Study the drawing (mm; zero at the part's minimum x, y, z) and answer. A direction names the side the tool comes from. Coordinates: 2 decimals unless noted, no trailing zeros. Loops run counter-clockwise (first coordinate to the right, second up) from the corner with the lowest first, then second, coordinate; pieces in that order, holes last. Notation, with made-up numbers: (-26.75, -31) - (-0.75, -31) arc R18 ccw to (-0.75, -16) - close; hole circle Ø8 at (41.25, -28.5). An arc over 180 degrees is marked (long way). Use one line per item in the form item = value. Start each with the question number.
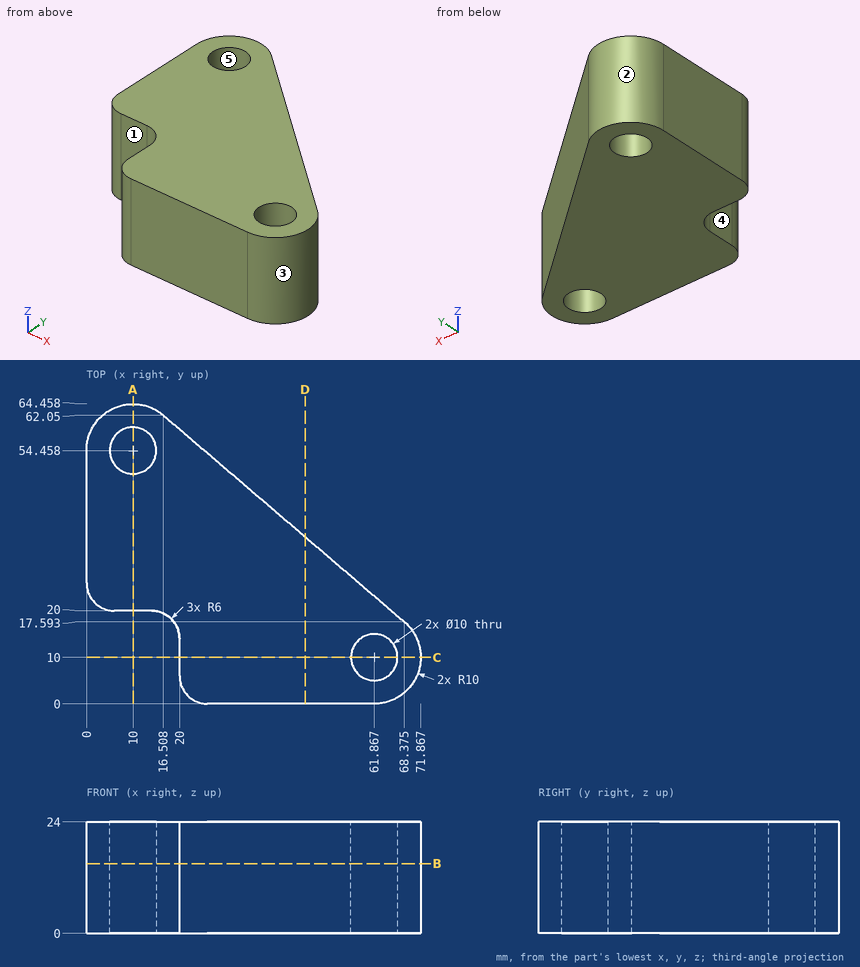
(1) For the marked faces 1 and 2, determine the directions among +Z, -Z, +X, -X, +Y, -Y from which every point of the face is accessible in a straight line to the end or side of a thin tool.
(2) Each of these flat-tipped pins is pushed along its axis until it touches: pin 1 Ø4 at (y, z) = (7, 3.5) entering from +X; pin 2 Ø16 at (x, y) = (61.87, 10) entering from -Z; pin 3 Ø9 at (x, z) = (11, 9) entering from -Y; pin 4 Ø6 at (x, y) = (10, 54.46) entering from +Z. Where does it stop, or does it pass through?
(3) A cutting plane is placed at A-A (x = 10). Determine the outline of the cut face in (y, z).
(4) Determine the mould class of the marked faces 3, 4 and 5 for opening direction Y: +Y half, -Y half, draft (parallel to the pull), parting line (faces both ways), or undercut.
(5) A cutting plane is placed at C-C (y = 10). Determine the outline of the cut face in (x, z), then the cut area to 3 significant figures.
(6) Find the intervals of material crossed by probe 1 along Y at (x, z) = (10, 16.5); probe 2 along X at (y, z) = (59, 19) (1 decimal); probe 3 along X at (y, z) = (45, 9.5), in increasing order. Write a range as from..to.
(7) A cutting plane is placed at D-D (x = 47). Determine the outline of the cut face in (y, z) (1 decimal), then the cut area to 3 significant figures.
(8) A cutting plane is placed at B-B (z = 15). State how many separate pieces and enclosed holes the cut face has, then the cut area to 3 significant figures.
Evaluation:
q1.face_1 = +Z, -Z, -X, -Y
q1.face_2 = +Z, -Z, +Y
q2.pin_1 = 71.82
q2.pin_2 = 0
q2.pin_3 = 19.81
q2.pin_4 = through
q3.outline = (20, 0) - (49.46, 0) - (49.46, 24) - (20, 24) - close; (59.46, 0) - (64.46, 0) - (64.46, 24) - (59.46, 24) - close
q4.face_3 = parting line
q4.face_4 = draft
q4.face_5 = undercut
q5.outline = (20, 0) - (56.87, 0) - (56.87, 24) - (20, 24) - close; (66.87, 0) - (71.87, 0) - (71.87, 24) - (66.87, 24) - close
q5.area = 1,000 mm^2
q6.probe_1 = 20..49.46, 59.46..64.46
q6.probe_2 = 1.1..7.9, 12.1..20.1
q6.probe_3 = 0..36.4
q7.outline = (0, 0) - (35.9, 0) - (35.9, 24) - (0, 24) - close
q7.area = 862 mm^2
q8.separate_pieces = 1
q8.enclosed_holes = 2
q8.area = 2,570 mm^2
